```python
from build123d import *

# Parameters (mm, degrees)
F0_W      = 112.1267676353
F0_H      = 38.257420063
F1_DEPTH  = 137.870118022
F2_W      = 68.7767341733
F2_H      = 25.1477137208
F3_DEPTH  = 137.871118022
F4_R      = 2.38125
F5_DEPTH  = 112.1277676353
F6_R      = 2.38125
F7_DEPTH  = 112.1277676353
F9_DEPTH  = 112.1277676353
F11_DEPTH = 25.4
F12_W     = 68.58
F12_H     = 38.1
F13_DEPTH = 6.35


with BuildPart() as f1:
    # F0 (on Front) → F1 (new body)
    with BuildSketch(Plane.XZ):
        with Locations((-1.3227313757, 19.1287100315)):
            Rectangle(F0_W, F0_H)
    extrude(amount=F1_DEPTH)

    # F2 (on face) → F3 (cut, through all)
    with BuildSketch(Plane.XZ.offset(137.870118022)):
        with Locations((-0.8782893419, 12.5738568604)):
            Rectangle(F2_W, F2_H)
    extrude(amount=-F3_DEPTH, mode=Mode.SUBTRACT)

    # F4 (on face) → F5 (cut, through all)
    with BuildSketch(Plane.YZ.offset(54.740652442)):
        with Locations((-128.4904330969, 9.1332495213)):
            Circle(F4_R)
    extrude(amount=-F5_DEPTH, mode=Mode.SUBTRACT)

    # F6 (on face) → F7 (cut, through all)
    with BuildSketch(Plane.YZ.offset(54.740652442)):
        with Locations((-6.499979645, 4.1290447116)):
            Circle(F6_R)
    extrude(amount=-F7_DEPTH, mode=Mode.SUBTRACT)

    # F8 (on face) → F9 (cut, through all)
    with BuildSketch(Plane.YZ.offset(54.740652442)):
        with BuildLine():
            Line((-106.8989974441, 0), (-30.9711205779, 0))
            ThreePointArc((-30.9711205779, 0), (-68.935059011, 30.0939472481), (-106.8989974441, 0))
        make_face()
    extrude(amount=-F9_DEPTH, mode=Mode.SUBTRACT)

    # F10 (on face) → F11 (join)
    with BuildSketch(Plane.XY.offset(38.257420063)):
        Polygon((54.740652442, -91.2534669042), (0, -91.2534669042), (-57.3861151934, -91.2534669042), (-57.3861151934, -137.870118022), (54.740652442, -137.870118022), align=None)
    extrude(amount=F11_DEPTH)

    # F12 (on face) → F13 (cut)
    with BuildSketch(Plane.XY.offset(63.657420063)):
        with Locations((-16.6207363016, -115.6102344394)):
            Rectangle(F12_W, F12_H)
    extrude(amount=-F13_DEPTH, mode=Mode.SUBTRACT)


solid = f1.part
```
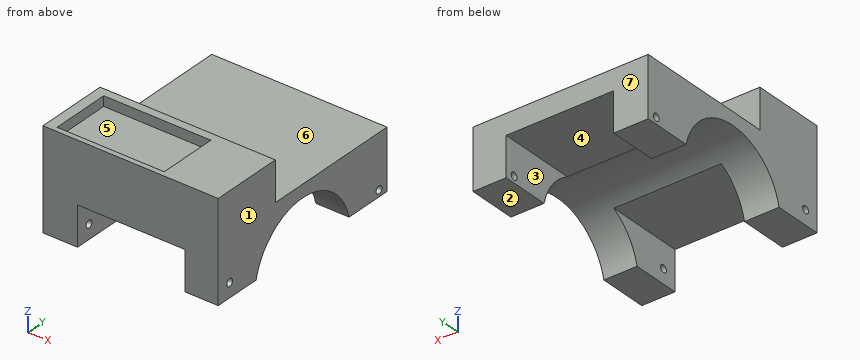
Input: part model. Units: mm. Frame: model coordinates. Face numbers are marked on the shaded views. A direction names the side the tool comes from. Give positions to 0.01 mm unless a question says otherwise; leave off trailing zeros. Order: outer loops, then holes, each group sorted by start corner. A loop starts at its lowest first (then second) coordinate and runs counter-clockwise, first axis right, second up.
1. Line query: probe 1 along X at (y, z) = (-29, 9); probe 2 along Y at (x, z) = (-15, 42); probe 3 along Z at (x, y) = (9, -7). Output: solid intervals per line, ascending.
Computed:
probe 1: x = -57.39 to -35.27, 33.51 to 54.74
probe 2: y = -137.87 to -91.25
probe 3: z = 25.15 to 38.26
2. Cut plane A-A (x = -20.5). Return loops of the section in (y, z), and give its area (3 significant figures).
Computed:
outline: (-137.87, 25.15) - (-87.94, 25.15) arc R38.99 cw to (-49.93, 25.15) - (0, 25.15) - (0, 38.26) - (-91.25, 38.26) - (-91.25, 63.66) - (-96.56, 63.66) - (-96.56, 57.31) - (-134.66, 57.31) - (-134.66, 63.66) - (-137.87, 63.66) - close
area: 2,620 mm2
3. Set-up query: the marked faces 4, 5, 6 and 7. Return all of +Z, -Z, +X, -X, +Y, -Y with unobstructed straight access to the full face (end or side cutting, diameter ignored); none if empty.
Computed:
face 4: -Z, +Y, -Y
face 5: +Z
face 6: +Z, +X, -X, +Y
face 7: +Z, -Z, +X, -X, +Y
4. Cut plane D-D (x = -49). Return loops of the section in (y, z), and give its area (3 significant figures).
Computed:
outline: (-137.87, 0) - (-106.9, 0) arc R38.99 cw to (-30.97, 0) - (0, 0) - (0, 38.26) - (-91.25, 38.26) - (-91.25, 63.66) - (-96.56, 63.66) - (-96.56, 57.31) - (-134.66, 57.31) - (-134.66, 63.66) - (-137.87, 63.66) - close; hole circle Ø4.76 at (-128.49, 9.13); hole circle Ø4.76 at (-6.5, 4.13)
area: 4,480 mm2
5. Cut plane B-B (z = 28). Return loops of the section in (x, y), and give its area (3 significant figures).
Computed:
outline: (-57.39, -137.87) - (54.74, -137.87) - (54.74, -81.54) - (-57.39, -81.54) - close; (-57.39, -56.33) - (54.74, -56.33) - (54.74, 0) - (-57.39, 0) - close
area: 12,600 mm2
6. Draft query along X for the marked faces 1, 2 and 3. Return one class per face: released by +X, released by -X, zero draft, split by the parting line, or undercut.
Computed:
face 1: released by +X
face 2: zero draft
face 3: undercut
7. Cut plane C-C (y = -128.5). Return loops of the section in (x, z), and give its area (3 significant figures).
Computed:
outline: (-57.39, 0) - (-35.27, 0) - (-35.27, 6.75) - (-57.39, 6.75) - close; (-57.39, 11.51) - (-35.27, 11.51) - (-35.27, 25.15) - (33.51, 25.15) - (33.51, 11.51) - (54.74, 11.51) - (54.74, 63.66) - (17.67, 63.66) - (17.67, 57.31) - (-50.91, 57.31) - (-50.91, 63.66) - (-57.39, 63.66) - close; (33.51, 0) - (54.74, 0) - (54.74, 6.75) - (33.51, 6.75) - close
area: 4,770 mm2
8. Pin query (flat end, axial travel): pin 1 Ø4 at (y, z) = (-128.49, 9.13) entering from +X; pin 2 Ø12.5 at (x, z) = (-26, 47) entering from +Y; pin 3 Ø15 at (x, y) = (7.5, -32) entering from -Z; pin 4 Ø10 at (x, y) = (-45.5, -38) entering from +Z. Return the tip coordinate at first contact, or that it passes through.
Computed:
pin 1: passes through
pin 2: stops at y = -91.25
pin 3: stops at z = 25.15
pin 4: stops at z = 38.26
